Design review of the part built by this model. Coordinates are the model's own, in mm. Face numbers are marked on the shaded views. A direction names the side the tool comes from. Round coordinates to 2 decimals unless told otherwise and drop trailing zeros. Write each loop counter-clockwise with the first axis right and the second up, starting at its lowest first coordinate (ties: lowest second). Pieces come first, ordered by that corner, then holes. Notation, with made-up numbers: (88.5, 37) - (111.5, 37) arc R37 cw to (111.5, 74) - close; hole circle Ø5 at (42.5, 18). An arc over 180 degrees is marked (long way). Use one line per item in the form item = value.
```python
from build123d import *

# Parameters (mm, degrees)
SKETCH2_W           = 75
SKETCH2_H           = 32
BOSS_EXTRUDE2_DEPTH = 3.102863873
SKETCH4_W           = 6.1
SKETCH4_H           = 9.4
SKETCH4_R           = 1.9
BOSS_EXTRUDE4_DEPTH = 1.095
SKETCH7_W           = 14.8
SKETCH7_H           = 32
TRIM_DEPTH          = 69.646631381
SKETCH8_W           = 6.1
SKETCH8_H           = 11.621856523
BOSS_EXTRUDE6_DEPTH = 3.102863873
SKETCH5_W           = 6.1
SKETCH5_H           = 9.4
SKETCH5_R           = 1.9
BOSS_EXTRUDE5_DEPTH = 3
SKETCH9_R           = 1.9
BOSS_EXTRUDE8_DEPTH = 3
SKETCH10_W          = 20
SKETCH10_H          = 40
BOSS_EXTRUDE9_DEPTH = 4
SKETCH11_R          = 1.9
CUT_EXTRUDE2_DEPTH  = 4


with BuildPart() as part:
    # Sketch2 → Boss-Extrude2 (new body)
    with BuildSketch(Plane(origin=(0, -5, 0), x_dir=(-1, 0, 0), z_dir=(0, -1, 0))):
        with Locations((-22.5, 16)):
            Rectangle(SKETCH2_W, SKETCH2_H)
    extrude(amount=-BOSS_EXTRUDE2_DEPTH)

    # Sketch4 → Boss-Extrude4 (add)
    # profile 1 of 2: a face of its own
    with BuildSketch(Plane(origin=(0, 0, -30.905), x_dir=(-1, 0, 0), z_dir=(0, 0, -1))):
        with Locations((-8.05, 2.802863873)):
            Rectangle(SKETCH4_W, SKETCH4_H)
        with Locations((-8.05, 3.602863873)):
            Circle(SKETCH4_R, mode=Mode.SUBTRACT)
    # profile 2 of 2: a face of its own
    with BuildSketch(Plane(origin=(0, 0, -30.905), x_dir=(-1, 0, 0), z_dir=(0, 0, -1))):
        with Locations((-42.15, 2.802863873)):
            Rectangle(SKETCH4_W, SKETCH4_H)
        with Locations(Location((-42.15, 3.602863873, 0), (0, 0, 180))):
            Circle(SKETCH4_R, mode=Mode.SUBTRACT)
    extrude(amount=BOSS_EXTRUDE4_DEPTH)

    # Sketch7 → trim (cut, through all)
    with BuildSketch(Plane(origin=(0, -1.897136127, 0), x_dir=(1, 0, 0), z_dir=(0, 1, 0))):
        with Locations((52.6, 16)):
            Rectangle(SKETCH7_W, SKETCH7_H)
    extrude(amount=-TRIM_DEPTH, mode=Mode.SUBTRACT)

    # Sketch8 → Boss-Extrude6 (add)
    with BuildSketch(Plane(origin=(0, -1.897136127, 0), x_dir=(1, 0, 0), z_dir=(0, 1, 0))):
        with Locations((33.76, -5.810928261)):
            Rectangle(SKETCH8_W, SKETCH8_H)
    extrude(amount=-BOSS_EXTRUDE6_DEPTH)

    # Sketch5 → Boss-Extrude5 (add)
    with BuildSketch(Plane.XY.offset(11.621856523)):
        with Locations((33.76, 2.802863873)):
            Rectangle(SKETCH5_W, SKETCH5_H)
        with Locations((33.76, 3.602863873)):
            Circle(SKETCH5_R, mode=Mode.SUBTRACT)
    extrude(amount=-BOSS_EXTRUDE5_DEPTH)

    # Sketch9 → Boss-Extrude8 (add)
    # profile 1 of 2: a face of its own
    with BuildSketch(Plane(origin=(0, 0, -32), x_dir=(-1, 0, 0), z_dir=(0, 0, -1))):
        Polygon((-45.2, 7.502863873), (-39.1, 7.502863873), (-39.1, -1.897136127), (-39.1, -5), (-45.2, -5), align=None)
        with Locations(Location((-42.15, 3.602863873, 0), (0, 0, 180))):
            Circle(SKETCH9_R, mode=Mode.SUBTRACT)
    # profile 2 of 2: a face of its own
    with BuildSketch(Plane(origin=(0, 0, -32), x_dir=(-1, 0, 0), z_dir=(0, 0, -1))):
        Polygon((-11.1, -1.897136127), (-11.1, 7.502863873), (-5, 7.502863873), (-5, -1.897136127), (-5, -5), (-11.1, -5), align=None)
        with Locations((-8.05, 3.602863873)):
            Circle(SKETCH9_R, mode=Mode.SUBTRACT)
    extrude(amount=BOSS_EXTRUDE8_DEPTH)

    # Sketch10 → Boss-Extrude9 (add)
    with BuildSketch(Plane(origin=(0, -1.897136127, 0), x_dir=(1, 0, 0), z_dir=(0, 1, 0))):
        with Locations((-10, 15.4525)):
            Rectangle(SKETCH10_W, SKETCH10_H)
    extrude(amount=-BOSS_EXTRUDE9_DEPTH)

    # Sketch11 → Cut-Extrude2 (cut)
    with BuildSketch(Plane(origin=(0, -1.897136127, 0), x_dir=(1, 0, 0), z_dir=(0, 1, 0))):
        with Locations(Location((-15, 27.9525, 0), (0, 0, 270))):
            Circle(SKETCH11_R)
        with Locations(Location((-5, 27.9525, 0), (0, 0, 270))):
            Circle(SKETCH11_R)
        with Locations(Location((-15, 2.9525, 0), (0, 0, 270))):
            Circle(SKETCH11_R)
        with Locations(Location((-5, 2.9525, 0), (0, 0, 270))):
            Circle(SKETCH11_R)
    extrude(amount=-CUT_EXTRUDE2_DEPTH, mode=Mode.SUBTRACT)


solid = part.part
```
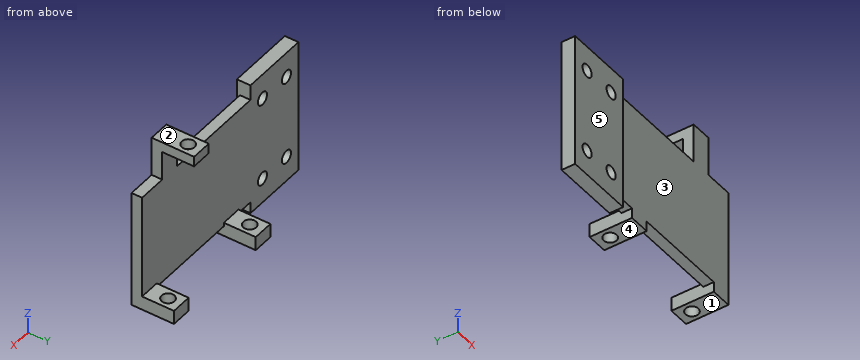
Q1. We need section A-A on x = 42.15. Write out the cut boundary in (y, z) (3 decimals), then the cut area to 3 significant figures.
Calculated:
outline = (-5, -35) - (1.703, -35) - (1.703, -30.905) - (-1.897, -30.905) - (-1.897, 0) - (-5, 0) - close; (5.503, -35) - (7.503, -35) - (7.503, -30.905) - (5.503, -30.905) - close
area = 132 mm2
Q2. For P1, Ø1.6, axis at x = 18, y = -3.5, coming from the +Z side; P2, Ø1.2, axis at y = 3, z = -33.5, coming from the -X side; P3, Ø12, axis at x = 14.5, z = -14, coming from the -Y side, all flat-tipped, find the tip position at first contact; note any pin that passes through.
Calculated:
P1 = 0
P2 = 5
P3 = -5
Q3. To check wall thickness, follow line 1 along Y through (x, z) = (33.76, 9.65); line 2 along X through (y, z) = (5, -31); line 3 along Z through (x, y) = (6, 5.25) (3 decimals). State the ranges of each line that lie inside material, in increasing order. Write a range as from..to.
Calculated:
line_1 = -5..1.7, 5.5..7.5
line_2 = 5..6.76, 9.34..11.1, 39.1..40.86, 43.44..45.2
line_3 = -35..-30.905
Q4. We need section C-C on y = 6.25. Write out the cut boundary in (x, z) (3 decimals), then the cut area to 3 significant figures.
Calculated:
outline = (5, -35) - (11.1, -35) - (11.1, -30.905) - (5, -30.905) - close; (30.71, 8.622) - (36.81, 8.622) - (36.81, 11.622) - (30.71, 11.622) - close; (39.1, -35) - (45.2, -35) - (45.2, -30.905) - (39.1, -30.905) - close
area = 68.3 mm2
Q5. Draft analysis for pull direction Y (two halves, no side actions). For the marked faces 4 and 5, state which applies: released by +Y, released by -Y, zero draft, split by the parting line, or undercut.
Calculated:
face_4 = zero draft
face_5 = released by -Y
Q6. We need section D-D on z = -7. Write out the cut boundary in (x, y), then the cut area to 3 significant figures.
Calculated:
outline = (-20, -5.9) - (0, -5.9) - (0, -5) - (45.2, -5) - (45.2, -1.9) - (-20, -1.9) - close
area = 220 mm2
Q7. We need section B-B on x = -15. Write out the cut boundary in (y, z).
Calculated:
outline = (-5.9, -35.45) - (-1.9, -35.45) - (-1.9, -29.85) - (-5.9, -29.85) - close; (-5.9, -26.05) - (-1.9, -26.05) - (-1.9, -4.85) - (-5.9, -4.85) - close; (-5.9, -1.05) - (-1.9, -1.05) - (-1.9, 4.55) - (-5.9, 4.55) - close
Q8. Machinability: for the marked faces 1, 2 and 3, which of the approach directions +Z, -Z, +X, -X, +Y, -Y give a long, thin tool a straight path to every point of the face, cutting with its end or side? Answer none if there is none.
Calculated:
face_1 = -Z, +X, +Y, -Y
face_2 = +Z, +X, -X, +Y, -Y
face_3 = +Z, -Z, +X, -Y
